Could you check a few things on this drawing? It's one solid part, dimensions in mm from its lowest x, y, z. A direction names the side the tool comes from. Coordinates: 2 decimals unless noted, no trailing zeros. Order: outer loops, then holes, each group sorted by start corner. A loop starts at its lowest first (then second) coordinate and runs counter-clockwise, first axis right, second up.
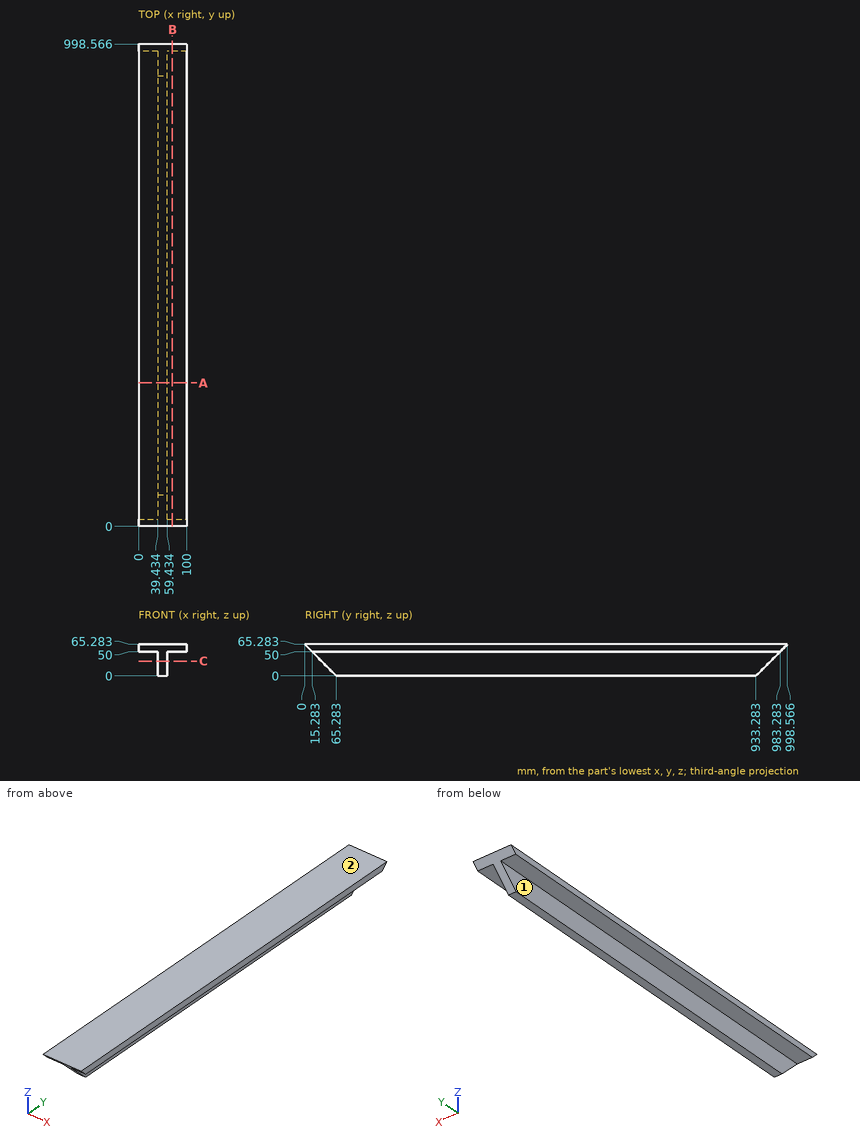
1. Imagine slicing it at C-C on z = 31. Please give me the cut outline in (x, y), then the cut area to 3 significant figures.
Completed:
outline: (39.43, 34.28) - (59.43, 34.28) - (59.43, 964.28) - (39.43, 964.28) - close
area: 18,600 mm2
2. Imagine slicing it at A-A on y = 297. Please give me the cut outline in (x, z).
Completed:
outline: (0, 50) - (39.43, 50) - (39.43, 0) - (59.43, 0) - (59.43, 50) - (100, 50) - (100, 65.28) - (0, 65.28) - close
3. Please list where these lines run through material, in increasing order: probe 1 along X at (y, z) = (169, 26); probe 2 along Z at (x, y) = (21.5, 91); probe 3 along Y at (x, z) = (44.5, 50).
Completed:
probe 1: x = 39.43 to 59.43
probe 2: z = 50 to 65.28
probe 3: y = 15.28 to 983.28
4. Imagine slicing it at B-B on x = 70. Please give me the cut outline in (y, z).
Completed:
outline: (0, 65.28) - (15.28, 50) - (983.28, 50) - (998.57, 65.28) - close
5. I'm going to push flat-ended pins straight in: pin 1 (8 mm diameter, centred on x = 60.5, z = 24, fed in from +Y); pin 2 (12 mm diameter, centred on x = 19, y = 313, fed in from -Z); pin 3 (8 mm diameter, centred on x = 42, z = 31.5, fed in from +Y). Where does each tip first touch, or does it pass through?
Completed:
pin 1: stops at y = 961.14
pin 2: stops at z = 50
pin 3: stops at y = 968.78
6. On a 3-axis mill with a long thin cutter (end or side, diameter ignored), from which of +Z, -Z, +X, -X, +Y, -Y can I reach the whole of each face in a straight line? I mean the marked faces 1 and 2. Say none if no direction works.
Completed:
face 1: -Z, -X, +Y, -Y
face 2: +Z, +X, -X, +Y, -Y
